Autodesk Inventor part; units mm, degrees
ref_plane "YZ Plane" through (0, 0, 0) normal (1, 0, 0) x (0, 1, 0)
ref_plane "XZ Plane" through (0, 0, 0) normal (0, 1, 0) x (-1, 0, 0)
ref_plane "XY Plane" through (0, 0, 0) normal (0, 0, 1) x (1, 0, 0)
sketch "スケッチ3" plane through (0, 0, 0) normal (1, 0, 0) x (0, 1, 0)
  line L0 (0, 0) -> (10.9667, 0)
  line L1 (10.9667, 0) -> (10.9667, -26)
  line L2 (10.9667, -26) -> (0, -26)
  line L3 (0, -26) -> (0, 0)
  line L4 (10.9667, 0) -> (6.9667, 0)
  line L5 (6.9667, 0) -> (6.9667, -26)
  line L6 (6.9667, -26) -> (10.9667, -26)
  line L7 (10.9667, -26) -> (10.9667, 0)
  line L8 (6.9667, 0) -> (0, -26)
  point P0 (6.9667, 0)
  dimension "d3" = 26
  dimension "d4" = 4
  dimension "d5" = 15
extrude "押し出し2" add sketch "スケッチ3" along normal blind 26 contours L0 L1 L2 L5 | L5 L2 L8
sketch "スケッチ4" plane through (0, 6.9667, 0) normal (0, 0, 1) x (1, 0, 0)
  line L0 (0, 4) -> (0, 0)
  line L1 (0, 0) -> (26, 0)
  line L2 (26, 4) -> (26, 0)
  line L3 (0, 4) -> (26, 4)
  circle A0 centre (5, 2) radius 0.8
  circle A1 centre (21, 2) radius 0.8
  point P0 (0, -6.9667)
  point P1 (0, 2)
  dimension "d8" = 1.6
  dimension "d9" = 1.6
  dimension "d10" = 5
  dimension "d11" = 5
extrude "押し出し8" cut sketch "スケッチ4" against normal through all contours A0 | A1
sketch "スケッチ8" plane through (26, 0, 0) normal (1, 0, 0) x (0, 0, -1)
  line L0 (26, 0) -> (26, 10.9667)
  line L1 (0, 6.9667) -> (26, 0)
  line L2 (26, 0) -> (0.8859, 6.7293)
  line L3 (0.8859, 6.7293) -> (-1.7023, -2.93)
  line L4 (-1.7023, -2.93) -> (23.4118, -9.6593)
  line L5 (23.4118, -9.6593) -> (26, 0)
  point P0 (0, 0)
  dimension "d39" = 26
  dimension "d40" = 10
extrude "押し出し9" add sketch "スケッチ8" against normal up to surface (26 mm away)
sketch "スケッチ5" plane through (26, 0, 0) normal (1, 0, 0) x (0, 0, -1)
  line L0 (0, 6.9667) -> (26, 0)
  line L1 (26, 0) -> (0.8859, 6.7293)
  line L2 (0.8859, 6.7293) -> (1.9212, 10.593)
  line L3 (1.9212, 10.593) -> (27.0353, 3.8637)
  line L4 (27.0353, 3.8637) -> (26, 0)
  circle A0 centre (21.688, 3.2259) radius 0.8
  circle A1 centre (6.2332, 7.3671) radius 0.8
  line L5 (-1.7023, -2.93) -> (-0.667, 0.9337)
  line L6 (-0.667, 0.9337) -> (24.4471, -5.7956)
  line L7 (24.4471, -5.7956) -> (23.4118, -9.6593)
  line L8 (23.4118, -9.6593) -> (-1.7023, -2.93)
  line L9 (-1.7023, -2.93) -> (23.4118, -9.6593)
  circle A2 centre (3.645, -2.2922) radius 0.8
  circle A3 centre (19.0998, -6.4333) radius 0.8
  point P0 (0, 0)
  dimension "d14" = 4
  dimension "d15" = 26
  dimension "d16" = 1.6
  dimension "d17" = 1.6
  dimension "d18" = 2
  dimension "d19" = 2
  dimension "d20" = 5
  dimension "d21" = 5
  dimension "d43" = 1.6
  dimension "d44" = 1.6
  dimension "d45" = 2
  dimension "d46" = 2
  dimension "d47" = 5
  dimension "d48" = 5
extrude "押し出し4" cut sketch "スケッチ5" against normal through all contours A0 | A1 | A2 | A3
equation "\"d18\" = d19"
equation "\"d45\" = d19"
equation "\"d46\" = d19"
equation "\"d47\" = d20"
equation "\"d48\" = d21"
properties part number "arm_middle"
Design review of the part built by this model. Coordinates are the model's own, in mm. A direction names the side the tool comes from. Give positions to 0.01 mm unless a question says otherwise; leave off trailing zeros. Loops run counter-clockwise (first coordinate to the right, second up) from the corner with the lowest first, then second, coordinate; pieces in that order, holes last. Notation, with made-up numbers: M 64,-35.5 L 79,-35.5 A17 cw 79,-21.5 Z; hole C 12,20 d9. An arc over 180 degrees is marked long. Return JSON: item names as keys, results as strings. Group by question number.
Item 1: Mouldability with a two-part tool opening along Y and no side actions: class faces 1 (the flat face through (12.82, 6.85, -0.44)), 2 (the flat face through (13, 6, -26)), 3 (the flat face through (13, 10.967, -13)) as released by +Y, released by -Y, zero draft, split by the parting line, or undercut.
Item 2: We need section C-C (y = -4). Give the boundary of the cut face in (x, z).
Item 3: We need section A-A (x = 19.5). Give the boundary of the cut face in (y, z) (3 decimals).
Item 4: For probe 1 along Z at (x, y) = (4.5, 3); probe 2 along Y at (x, z) = (3.5, -19.5); probe 3 along Z at (x, y) = (5.25, 3.75), list the stretches that pass through material, from the lowest coordinate up.
Item 5: Tool access review of faces 4 (the cylindrical face through (13.18, 3.77, -21.1)), 5 (the flat face through (13, 9, 0)), 6 (the flat face through (13.18, 1.97, 0.39)): name each direction out of +Z, -Z, +X, -X, +Y, -Y from which nothing blocks a thin tool from reaching the whole face with its end or side.
Item 6: We need section B-B (y = 5.75). Give the boundary of the cut face in (x, z).
Item 7: Insertion check: pin 1 Ø12 at (x, y) = (11.5, -1) entering from +Z; pin 2 Ø1.3 at (y, z) = (7.37, -6.23) entering from -X; pin 3 Ø2.5 at (y, z) = (-2.29, -3.64) entering from -X; pin 4 Ø1 at (x, y) = (4, 9) entering from +Z. Each pin has a flat end and moves straight along its axis. Give the tip position at first contact, or say it passes through.
Output:
{
 "1": {"face 1": "undercut", "face 2": "zero draft", "face 3": "released by +Y"},
 "2": {"outline": "M 0,-24.93 L 26,-24.93 L 26,-2.29 L 0,-2.29 Z"},
 "3": {"outline": "M -9.659,-23.412 L 0,-26 L 10.967,-26 L 10.967,0 L 6.967,0 L 6.729,-0.886 L -2.93,1.702 Z; hole C -6.433,-19.1 d1.6; hole C -2.292,-3.645 d1.6; hole C 3.226,-21.688 d1.6; hole C 7.367,-6.233 d1.6"},
 "4": {"probe 1": "z = -26 to -22.46, -20.92 to 0.11", "probe 2": "y = -8.61 to -7.13, -5.74 to 10.97", "probe 3": "z = -26 to -22.29, -21.08 to -0.09"},
 "5": {"face 4": "+X, -X", "face 5": "+Z, +X, -X, +Y", "face 6": "+Z, +X, -X"},
 "6": {"outline": "M 0,-26 L 26,-26 L 26,-0.62 L 0,-0.62 Z"},
 "7": {"pin 1": "stops at z = 1.7", "pin 2": "passes through", "pin 3": "stops at x = 0", "pin 4": "stops at z = 0"}
}
